Can you work these out from the model? Positions are in its coordinate system, mm. Round coordinates to 2 decimals unless told otherwise and drop trailing zeros. Write each loop counter-clockwise with the first axis right and the second up, starting at its lowest first coordinate (ties: lowest second). Pieces come first, ordered by that corner, then holes. Notation, with made-up numbers: (89, 16.5) -> (96, 16.5) arc R29 ccw to (96, 38.5) -> close; hole circle Ø2 at (88, -6.75). An arc over 180 degrees is marked (long way). Use CSV: the item, a comma, the result in double quotes.
Autodesk Inventor part; units mm, degrees
ref_plane "YZ Plane" through (0, 0, 0) normal (1, 0, 0) x (0, 1, 0)
ref_plane "XZ Plane" through (0, 0, 0) normal (0, 1, 0) x (-1, 0, 0)
ref_plane "XY Plane" through (0, 0, 0) normal (0, 0, 1) x (1, 0, 0)
sketch "Sketch1" plane through (0, 0, 0) normal (0, 0, 1) x (1, 0, 0)
  line L0 (-60, -70) -> (60, -70)
  line L1 (60, -70) -> (60, 70)
  line L2 (60, 70) -> (-60, 70)
  line L3 (-60, 70) -> (-60, -70)
  line L4 (-60, -70) -> (60, 70) construction
  line L5 (60, -70) -> (-60, 70) construction
  line L6 (-60, 0) -> (60, 0) construction
  circle A0 centre (-60, 70) radius 20
  line L7 (60, 26.6315) -> (-14.7466, -70)
  point P0 (0, 0)
  point P1 (0, 0)
  point P2 (-40, 70)
  point P3 (-60, 50)
  dimension "d0" = 120
  dimension "d1" = 140
  dimension "d16" = 40
extrude "Plate1" add sketch "Sketch1" along normal blind 2 contours L3 A0 L2 L1 L7 L0
sketch "Sketch2" plane through (0, 0, 0) normal (0, 0, -1) x (-1, 0, 0)
  line L0 (-40, 50) -> (160, 50) construction
  line L1 (160, 50) -> (160, 30) construction
  line L2 (160, 30) -> (-40, 30) construction
  line L3 (-40, 30) -> (-40, 50) construction
  line L4 (-60, 70) -> (40, 70)
  line L5 (-60, 26.6315) -> (-60, 70)
  point P0 (0, 0)
  point P1 (-48, 100)
  point P2 (60, 70)
  point P3 (-60, -70)
  point P4 (-50, 98)
  dimension "d6" = 200
  dimension "d9" = 20
  dimension "d10" = 20
  dimension "d11" = 20
mark "Mark1"
equation "\"d2\" = Thickness"
equation "\"BendReliefWidth\" = Thickness"
equation "\"BendReliefDepth\" = 0.5 * Thickness"
equation "\"CornerReliefSize\" = 4 * Thickness"
equation "\"MinimumRemnant\" = 2 * Thickness"
equation "\"TransitionRadius\" = BendRadius"
equation "\"JacobiRadiusSize\" = BendRadius"
equation "\"GapSize\" = Thickness"
properties part number "TRM 034 motor pillar" material "AISI 304"
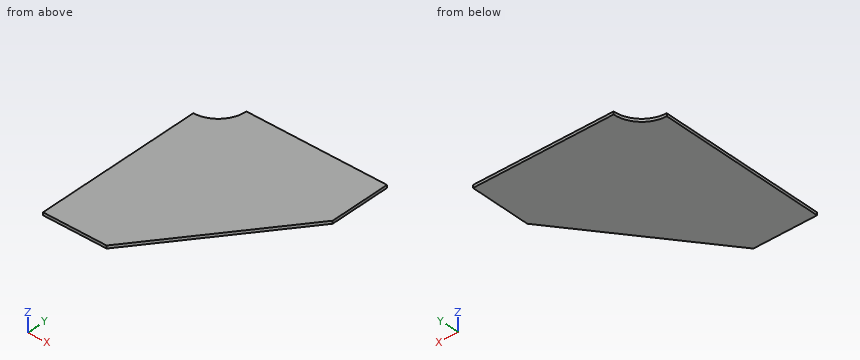
Q1. Please list where these lines run through material, in increasing order: probe 1 along Y at (x, z) = (-2.5, 0.3); probe 2 along X at (y, z) = (64, 0.85); probe 3 along X at (y, z) = (-62.5, 1.6).
Resolved:
probe 1,"y = -54.17 to 70"
probe 2,"x = -40.92 to 60"
probe 3,"x = -60 to -8.95"
Q2. Suppose I cut it at A-A (z = 0.4). Write out the boundary of the cut face in (x, y), and give its area (3 significant figures).
Resolved:
outline,"(-60, -70) -> (-14.75, -70) -> (60, 26.63) -> (60, 70) -> (-40, 70) arc R20 cw to (-60, 50) -> close"
area,"12,900 mm^2"
Q3. Suppose I cut it at C-C (x = 2.5). Write out the boundary of the cut face in (y, z), and give its area (3 significant figures).
Resolved:
outline,"(-47.7, 0) -> (70, 0) -> (70, 2) -> (-47.7, 2) -> close"
area,"235 mm^2"
Q4. Suppose I cut it at B-B (y = -59). Write out the boundary of the cut face in (x, z), and give its area (3 significant figures).
Resolved:
outline,"(-60, 0) -> (-6.24, 0) -> (-6.24, 2) -> (-60, 2) -> close"
area,"108 mm^2"
